Can you work these out from the model? Positions are in its coordinate system, mm. A direction names the side the tool comes from. Round coordinates to 2 decimals unless told otherwise and drop trailing zeros. Write each loop counter-clockwise with the first axis right and the second up, starting at its lowest first coordinate (ties: lowest second). Pieces come first, ordered by that corner, then holes. Notation, with made-up numbers: M 58,-27.5 L 67,-27.5 A18 ccw 67,-17.5 Z; hole C -36,-26 d9. An arc over 180 degrees is marked long. Use one line per item in the form item = value. Start each with the question number.
```python
from build123d import *

# Parameters (mm, degrees)
F0_R     = 177.8
F0_R_2   = 76.2
F1_DEPTH = 57.15
F2_R     = 76.2
F3_DEPTH = 31.75
F4_R     = 7.9375
F5_DEPTH = 63.5
F6_R     = 5.08


with BuildPart() as f1:
    # F0 (on Front) → F1 (new body, symmetric)
    with BuildSketch(Plane.XZ):
        Circle(F0_R)
        Circle(F0_R_2, mode=Mode.SUBTRACT)
    extrude(amount=F1_DEPTH, both=True)

    # F2 (on Front) → F3 (join, symmetric)
    with BuildSketch(Plane.XZ):
        Circle(F2_R)
    extrude(amount=F3_DEPTH, both=True)

    # F4 (on face) → F5 (cut, symmetric)
    with BuildSketch(Plane.XZ.offset(31.75)):
        Circle(F4_R)
    extrude(amount=F5_DEPTH, both=True, mode=Mode.SUBTRACT)

    # F6
    f6_edges = [f1.edges().sort_by_distance(p)[0] for p in [
        (-177.8, -57.15, 0),
        (-177.8, 57.15, 0),
    ]]
    fillet(f6_edges, radius=F6_R)


solid = f1.part
```
1. Please list where these lines run through material, in increasing order: line 1 along Z through (x, y) = (0, 1); line 2 along Z through (x, y) = (0, 38.5); line 3 along Y through (x, z) = (31, 66.5).
2. If we section it at B-B (x = 0): List the corners of the cut face in (y, z) for me.
3. Which directions (+Z, -Z, +X, -X, +Y, -Y) give clear straight access to the entire face, cutting with the end or side of a thin tool? Please do faces 1 (the face through (-60.47, -44.272, -46.367)), 2 (the face through (74, -57.15, -36)), 3 (the face through (-60.47, 44.628, -46.367)).
4. If we mould it in two halves opening along X, with no side actions, what happens to faces 4 (the face through (74, 57.15, -36)), 5 (the face through (-1.72, -0.44, -7.75)), 6 (the face through (169.59, -0.73, 53.41)), 7 (the face through (16, -31.75, 1))? For each: pulls with the +X half, pulls with the -X half, needs draft (parallel to the pull), parting line crosses it, or undercut.
5. If we section it at C-C (y = 27.5): List the corners of the cut face in (x, z) for me (1 decimal).
6. Will these pins go through, and if not, where does the flat tip stop? pin 1 (10 mm diameter, centred on y = -11.5, z = -78.5, fed in from -X); pin 2 (12 mm diameter, centred on y = -39, z = -91, fed in from -X); pin 3 (1.5 mm diameter, centred on x = -10.5, y = 6, fed in from +Z).
7. If we section it at A-A (z = 0): List the corners of the cut face in (x, y) for me.
Model answer:
q1.line_1 = -177.8 to -7.94, 7.94 to 177.8
q1.line_2 = -177.8 to -76.2, 76.2 to 177.8
q1.line_3 = -31.75 to 31.75
q2.outline = M -57.15,-172.72 A5.08 ccw -52.07,-177.8 L 52.07,-177.8 A5.08 ccw 57.15,-172.72 L 57.15,-76.2 L 31.75,-76.2 L 31.75,-7.94 L -31.75,-7.94 L -31.75,-76.2 L -57.15,-76.2 Z; M -57.15,76.2 L -31.75,76.2 L -31.75,7.94 L 31.75,7.94 L 31.75,76.2 L 57.15,76.2 L 57.15,172.72 A5.08 ccw 52.07,177.8 L -52.07,177.8 A5.08 ccw -57.15,172.72 Z
q3.face_1 = -Y
q3.face_2 = +Z, -Z, +X, -X, -Y
q3.face_3 = +Y
q4.face_4 = needs draft
q4.face_5 = undercut
q4.face_6 = parting line crosses it
q4.face_7 = undercut
q5.outline = C 0,0 d355.6; hole C 0,0 d15.9
q6.pin_1 = -161.9
q6.pin_2 = -156.17
q6.pin_3 = 177.53
q7.outline = M -177.8,-52.07 A5.08 ccw -172.72,-57.15 L -76.2,-57.15 L -76.2,-31.75 L -7.94,-31.75 L -7.94,31.75 L -76.2,31.75 L -76.2,57.15 L -172.72,57.15 A5.08 ccw -177.8,52.07 Z; M 7.94,-31.75 L 76.2,-31.75 L 76.2,-57.15 L 172.72,-57.15 A5.08 ccw 177.8,-52.07 L 177.8,52.07 A5.08 ccw 172.72,57.15 L 76.2,57.15 L 76.2,31.75 L 7.94,31.75 Z
